```python
from build123d import *

# Parameters (mm, degrees)
SKETCH1_W           = 297.73626
SKETCH1_H           = 182.7784
BOSS_EXTRUDE1_DEPTH = 15.24
CUT_EXTRUDE1_DEPTH  = 350.695698609
SKETCH4_W           = 91.3892
SKETCH4_H           = 15.24
CUT_EXTRUDE3_DEPTH  = 350.695698609
SKETCH5_W           = 297.73626
SKETCH5_H           = 79.467279424
BOSS_EXTRUDE2_DEPTH = 127
FILLET1_R           = 12.7
FILLET2_R           = 12.7
FILLET3_R           = 12.7
SKETCH6_R           = 26.104541014
BOSS_EXTRUDE3_DEPTH = 19.304
SKETCH7_R           = 20.913687516
BOSS_EXTRUDE4_DEPTH = 21.844
CHAMFER1_SIZE       = 10
SKETCH8_R           = 4.376446561
CUT_EXTRUDE4_DEPTH  = 21.844


with BuildPart() as part:
    # Sketch1 → Boss-Extrude1 (new body)
    with BuildSketch(Plane(origin=(0, 0, 0), x_dir=(1, 0, 0), z_dir=(0, 1, 0))):
        with Locations((148.86813, 91.3892)):
            Rectangle(SKETCH1_W, SKETCH1_H)
    extrude(amount=BOSS_EXTRUDE1_DEPTH)

    # Sketch2 → Cut-Extrude1 (cut, through all)
    with BuildSketch(Plane.ZY):
        with BuildLine():
            ThreePointArc((-43.45432, 0), (-56.15432, 12.7), (-68.85432, 0))
            Line((-68.85432, 0), (-43.45432, 0))
        make_face()
        with BuildLine():
            ThreePointArc((-113.92408, 0), (-126.62408, 12.7), (-139.32408, 0))
            Line((-139.32408, 0), (-126.62408, 0))
            Line((-126.62408, 0), (-113.92408, 0))
        make_face()
    extrude(amount=-CUT_EXTRUDE1_DEPTH, mode=Mode.SUBTRACT)

    # Sketch4 → Cut-Extrude3 (cut, through all)
    with BuildSketch(Plane.ZY):
        with Locations((-45.6946, 7.62)):
            Rectangle(SKETCH4_W, SKETCH4_H)
    extrude(amount=-CUT_EXTRUDE3_DEPTH, mode=Mode.SUBTRACT)

    # Sketch5 → Boss-Extrude2 (add)
    with BuildSketch(Plane(origin=(0, 15.24, 0), x_dir=(1, 0, 0), z_dir=(0, 1, 0))):
        with Locations((148.86813, 143.044760288)):
            Rectangle(SKETCH5_W, SKETCH5_H)
    extrude(amount=BOSS_EXTRUDE2_DEPTH)

    # Fillet1
    fillet1_edges = [part.edges().sort_by_distance(p)[0] for p in [
        (148.86813, 142.24, -103.311120576),
    ]]
    fillet(fillet1_edges, radius=FILLET1_R)

    # Fillet2
    fillet2_edges = [part.edges().sort_by_distance(p)[0] for p in [
        (148.86813, 142.24, -182.7784),
    ]]
    fillet(fillet2_edges, radius=FILLET2_R)

    # Fillet3
    fillet3_edges = [part.edges().sort_by_distance(p)[0] for p in [
        (0, 72.39, -103.311120576),
        (0, 138.520256121, -107.030864455),
        (0, 64.77, -182.7784),
        (0, 142.24, -143.044760288),
        (0, 138.520256121, -179.058656121),
    ]]
    fillet(fillet3_edges, radius=FILLET3_R)

    # Sketch6 → Boss-Extrude3 (add)
    with BuildSketch(Plane.ZY):
        with Locations(Location((-143.044760288, 98.490679768, 0), (0, 0, 180))):
            Circle(SKETCH6_R)
    extrude(amount=BOSS_EXTRUDE3_DEPTH)

    # Sketch7 → Boss-Extrude4 (add)
    with BuildSketch(Plane.ZY.offset(19.304)):
        with Locations((-143.044760288, 98.490679768)):
            Circle(SKETCH7_R)
    extrude(amount=BOSS_EXTRUDE4_DEPTH)

    # Chamfer1
    chamfer1_edges = [part.edges().sort_by_distance(p)[0] for p in [
        (-41.148, 98.490679768, -163.958447804),
    ]]
    chamfer(chamfer1_edges, length=CHAMFER1_SIZE)

    # Sketch8 → Cut-Extrude4 (cut)
    with BuildSketch(Plane.ZY.offset(41.148)):
        with Locations((-143.044760288, 98.490679768)):
            Circle(SKETCH8_R)
        Polygon((-150.144784592, 100.727732071), (-152.082128716, 99.609205919), (-152.082128716, 97.372153616), (-150.144784592, 96.253627465), (-148.207440468, 97.372153616), (-148.207440468, 99.609205919), align=None)
    extrude(amount=-CUT_EXTRUDE4_DEPTH, mode=Mode.SUBTRACT)


solid = part.part
```
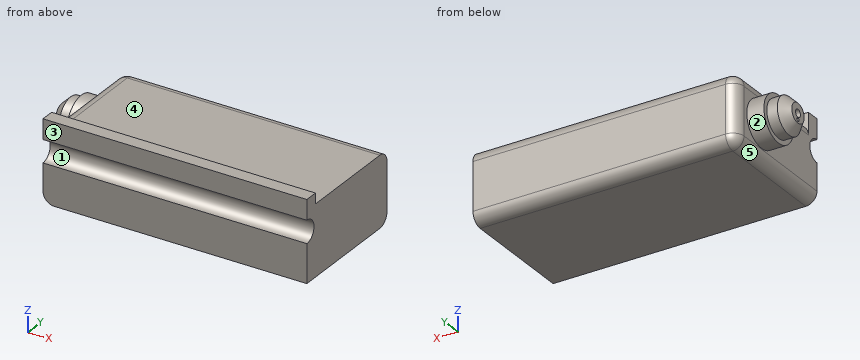
Model file for the job. Use its own axes, mm. Face numbers are marked on the shaded views. A direction names the side the tool comes from. Coordinates: 2 decimals unless noted, no trailing zeros. Write each loop counter-clockwise with the first axis right and the second up, starting at its lowest first coordinate (ties: lowest second). Pieces come first, ordered by that corner, then holes. Notation, with made-up numbers: (-19.5, 10.5) - (27.5, 10.5) arc R33 cw to (27.5, 42.5) - close; hole circle Ø10 at (-16, 87.5). An arc over 180 degrees is marked (long way). One line per item, written item: value. Start each with the question number.
1. Mould opens along Z. For the marked faces 1, 2 and 3 say: released by +Z, released by -Z, zero draft, split by the parting line, or undercut.
2. Slice it at D-D (z = -175). Write the cut outline in (x, y).
3. Slice it at A-A (x = 16). Write the cut outline in (y, z), plus the area to 3 significant figures.
4. Slice it at C-C (z = -109). Write the cut outline in (x, y).
5. Probe line 1 (Z direction, x = 111.5, y = 82.5); line 2 (X direction, y = 125, z = -118); line 3 (Y direction, x = 67.5, z = -98). List the from-to ranges inside material, lowest first. Write a range as from..to.
6. Tool access for the marked faces 4 and 5: list every direction of +Z, -Z, +X, -X, +Y, -Y with a clear straight run to the whole face (end or side of a thin tool).
7. Slice it at B-B (y = 42.5). Write the cut outline in (x, z), plus the area to 3 significant figures.
8. Flat gauge pins, fed straight in: pin 1 (2 mm diameter, centred on x = 66.5, y = 128, fed in from +Z); pin 2 (0.7 mm diameter, centred on x = -33, y = 98.5, fed in from +Z); pin 3 (0.7 mm diameter, centred on x = -27.5, y = 99, fed in from -Z). Where does each tip first touch, or does it go through?
Answers below:
1. face 1: undercut
1. face 2: split by the parting line
1. face 3: zero draft
2. outline: (0.99, 0) - (297.74, 0) - (297.74, 141.25) - (12.7, 141.25) arc R11.71 ccw to (0.99, 129.54) - close
3. outline: (0, -182.78) - (129.54, -182.78) arc R12.7 ccw to (142.24, -170.08) - (142.24, -116.01) arc R12.7 ccw to (129.54, -103.31) - (15.24, -103.31) - (15.24, -91.39) - (0, -91.39) - (0, -113.92) arc R12.7 cw to (0, -139.32) - close
3. area: 11,200 mm^2
4. outline: (0, 0) - (297.74, 0) - (297.74, 140.13) - (12.7, 140.13) arc R10.59 ccw to (2.11, 129.54) - (2.11, 15.24) - (0, 15.24) - close
5. line 1: z = -182.78..-103.31
5. line 2: x = 0..297.74
5. line 3: y = 0..15.24
6. face 4: +Z, +X, -X, +Y
6. face 5: -Z, -X, +Y, -Y
7. outline: (0, -170.08) arc R12.7 ccw to (12.7, -182.78) - (297.74, -182.78) - (297.74, -103.31) - (12.7, -103.31) arc R12.7 ccw to (0, -116.01) - close
7. area: 23,600 mm^2
8. pin 1: stops at z = -103.31
8. pin 2: stops at z = -123.63
8. pin 3: stops at z = -163.96
